from build123d import *

# Parameters (mm, degrees)
CUT_EXTRUDE_START        = -40
SKETCH_2_OUTSIDE_W       = 54.89
SKETCH_2_OUTSIDE_H       = 54.89
SKETCH_2_OUTSIDE_W_2     = 20
SKETCH_2_OUTSIDE_H_2     = 16
CUT_EXTRUDE_1_DEPTH      = 12
CUT_EXTRUDE_2_DEPTH      = 196.51214796
CUT_EXTRUDE_2_DEPTH_BACK = 196.51214796
SKETCH_3_R               = 2


with BuildPart() as part:
    # Эскиз1 → Повернуть1 (revolve)
    with BuildSketch(Plane.XY, mode=Mode.PRIVATE) as revolve_1_sk:
        Polygon((-6, 1), (-5, 0), (0, 0), (0, 162), (-8, 162), (-10, 160), (-10, 34), (-8, 32), (-8, 14), (-6, 12), align=None)
    revolve(revolve_1_sk.sketch.rotate(Axis((0, 0, 0), (0, 1, 0)), 270), axis=Axis((0, 0, 0), (0, 1, 0)))

    # Эскиз2 outside → Вырез-Вытянуть1 (cut)
    with BuildSketch(Plane(origin=(0, 162, 0), x_dir=(1, 0, 0), z_dir=(0, 1, 0)).offset(CUT_EXTRUDE_START)):
        Rectangle(SKETCH_2_OUTSIDE_W, SKETCH_2_OUTSIDE_H)
        Rectangle(SKETCH_2_OUTSIDE_W_2, SKETCH_2_OUTSIDE_H_2, mode=Mode.SUBTRACT)
    extrude(amount=-CUT_EXTRUDE_1_DEPTH, mode=Mode.SUBTRACT)

    # Эскиз3 → Вырез-Вытянуть2 (cut, two sides: drawn at the far end of the back side and taken through both)
    with BuildSketch(Plane(origin=(0, -33, 0), x_dir=(0.027583216315568815, 0, -0.9996195107027916), z_dir=(0.9996195107027916, 0, 0.027583216315568815)).offset(-CUT_EXTRUDE_2_DEPTH_BACK)):
        with Locations((0, 56)):
            Circle(SKETCH_3_R)
    extrude(amount=CUT_EXTRUDE_2_DEPTH + CUT_EXTRUDE_2_DEPTH_BACK, mode=Mode.SUBTRACT)


solid = part.part
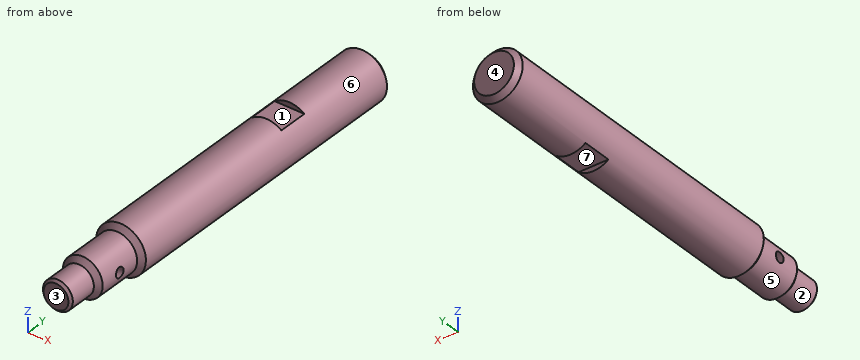
Build history of the part. All positions in model axes, mm. Face numbers are marked on the shaded views. A direction names the side the tool comes from. Round coordinates to 2 decimals unless told otherwise and drop trailing zeros. Order: outer loops, then holes, each group sorted by start corner. A loop starts at its lowest first (then second) coordinate and runs counter-clockwise, first axis right, second up. Notation, with made-up numbers: M 74,-4 L 128,-4 A23 cw 128,35 Z; hole C 33,21 d11. An arc over 180 degrees is marked long. Use CSV: the item, a comma, the result in double quotes. Start each with the question number.
(1) Drill centre lines: probe 1 along X at (y, z) = (20, 0); probe 2 along Z at (x, y) = (-0.25, 85); probe 3 along Y at (x, z) = (-3.75, 1.5). Where is each one in solid material? Low to high.
(2) Mould opens along Y. For the marked faces 1, 2, 3 and 4 say: +Y half, -Y half, draft (parallel to the pull), parting line (faces both ways), or undercut.
(3) Tool access for the marked faces 5, 6 and 7: list every direction of +Z, -Z, +X, -X, +Y, -Y with a clear straight run to the whole face (end or side of a thin tool).
(4) Flat gauge pins, fed straight in: P1, Ø1, axis at x = -1, z = 9, coming from the -Y side; P2, Ø10, axis at x = 7, y = 68, coming from the +Z side; P3, Ø3, axis at x = 6, y = 93, coming from the +Z side; P4, Ø10, axis at x = -4, z = -6.5, coming from the -Y side. Where does each tip first touch, or does it go through?
(5) Cut at B-B on y = 80. List the corners of the cut face in (x, z), then the cut area to 3 significant figures.
(6) Cut at A-A on y = 118. List the corners of the cut face in (x, z), then the cut area to 3 significant figures.
Findings:
1,probe 1,"x = -8 to 8"
1,probe 2,"z = -10 to 10"
1,probe 3,"y = 0 to 21.8, 24.2 to 162"
2,face 1,"undercut"
2,face 2,"draft"
2,face 3,"-Y half"
2,face 4,"+Y half"
3,face 5,"-Y"
3,face 6,"+Y, -Y"
3,face 7,"-Z, +X, -X"
4,P1,"stops at y = 32.56"
4,P2,"stops at z = 9.8"
4,P3,"stops at z = 8.93"
4,P4,"stops at y = 0"
5,outline,"C 0,0 d20"
5,area,"314 mm^2"
6,outline,"M -6,-8 L 6,-8 A10 ccw 6,8 L -6,8 A10 ccw Z"
6,area,"281 mm^2"
